from build123d import *

# Parameters (mm, degrees)
SKETCH_1_W      = 40
SKETCH_1_H      = 40.2
EXTRUDE_1_DEPTH = 2
SKETCH_2_W      = 1
SKETCH_2_H      = 40.2
EXTRUDE_2_DEPTH = 3


with BuildPart() as part:
    # 草图1 → 凸台-拉伸1 (new body)
    with BuildSketch(Plane(origin=(0, 0, 0), x_dir=(1, 0, 0), z_dir=(0, 1, 0))):
        Rectangle(SKETCH_1_W, SKETCH_1_H)
    extrude(amount=EXTRUDE_1_DEPTH)

    # 草图2 → 凸台-拉伸2 (add)
    with BuildSketch(Plane(origin=(0, 2, 0), x_dir=(1, 0, 0), z_dir=(0, 1, 0))):
        with Locations((-19.5, 0)):
            Rectangle(SKETCH_2_W, SKETCH_2_H)
        with Locations((-16.5, 0)):
            Rectangle(SKETCH_2_W, SKETCH_2_H)
        with Locations((-13.5, 0)):
            Rectangle(SKETCH_2_W, SKETCH_2_H)
        with Locations((-10.5, 0)):
            Rectangle(SKETCH_2_W, SKETCH_2_H)
        with Locations((-7.5, 0)):
            Rectangle(SKETCH_2_W, SKETCH_2_H)
        with Locations((-4.5, 0)):
            Rectangle(SKETCH_2_W, SKETCH_2_H)
        with Locations((-1.5, 0)):
            Rectangle(SKETCH_2_W, SKETCH_2_H)
        with Locations((1.5, 0)):
            Rectangle(SKETCH_2_W, SKETCH_2_H)
        with Locations((4.5, 0)):
            Rectangle(SKETCH_2_W, SKETCH_2_H)
        with Locations((7.5, 0)):
            Rectangle(SKETCH_2_W, SKETCH_2_H)
        with Locations((10.5, 0)):
            Rectangle(SKETCH_2_W, SKETCH_2_H)
        with Locations((13.5, 0)):
            Rectangle(SKETCH_2_W, SKETCH_2_H)
        with Locations((16.5, 0)):
            Rectangle(SKETCH_2_W, SKETCH_2_H)
        with Locations((19.5, 0)):
            Rectangle(SKETCH_2_W, SKETCH_2_H)
    extrude(amount=EXTRUDE_2_DEPTH)


solid = part.part
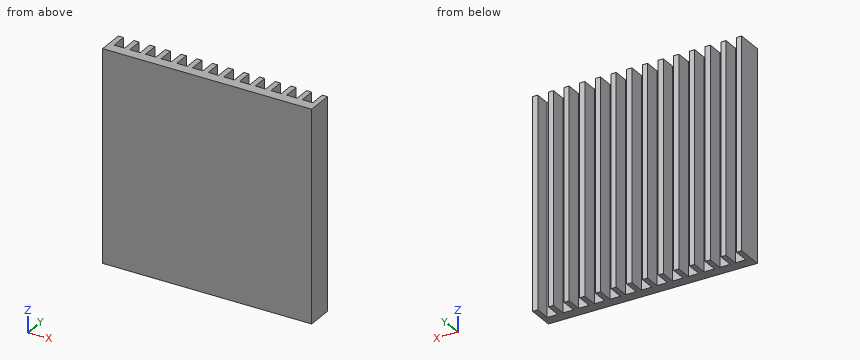
Read the model definition and answer for the solid it produces. Units are mm, in the model's axes. Round coordinates to 2 decimals unless told otherwise and drop trailing zeros. Loops run counter-clockwise (first coordinate to the right, second up) from the corner with the lowest first, then second, coordinate; pieces in that order, holes last. Notation, with made-up numbers: (51.5, -25) - (101.5, -25) arc R32 cw to (101.5, 10) - close; hole circle Ø8 at (24, 76.25). An arc over 180 degrees is marked (long way). One line per question, with ' | ' between items. Start each with the question number.
Q1. Section A-A on y = 3.7 is taken. Count the separate pieces of the cut face and the enclosed holes in it, plus the area to 3 significant figures.
Q2. Find the intervals of material crossed by L1, parallel to Y at x = 3.5, z = 7.5, in increasing order.
Q3. Section B-B on x = -6 is taken. Give the vertices of the cut face in (y, z), plus the area to 3 significant figures.
Q4. Flat-ended cylindrical pins translate along their axes: pin 1 (1.6 mm diameter, centred on x = 18.5, z = 4.5, fed in from +Y); pin 2 (0.6 mm diameter, centred on x = -8.5, z = -8, fed in from +Y). Find the tip coordinate at first contact, or state that the pin passes through.
Established:
1) separate pieces: 14 | enclosed holes: 0 | area: 563 mm²
2) L1: 0 to 2
3) outline: (0, -20.1) - (2, -20.1) - (2, 20.1) - (0, 20.1) - close | area: 80.4 mm²
4) pin 1: y = 5 | pin 2: y = 2
